from build123d import *

# Parameters (mm, degrees)
F0_W     = 130
F0_H     = 400
F0_R     = 5
F1_DEPTH = 4
F3_DEPTH = 5


with BuildPart() as f1:
    # F0 (on Right) → F1 (new body)
    with BuildSketch(Plane.YZ):
        with Locations((-28.497371, -1.37512)):
            Rectangle(F0_W, F0_H)
        with Locations((-63.497371, -21.37512)):
            Circle(F0_R, mode=Mode.SUBTRACT)
        with Locations((-13.497371, 168.62488)):
            Circle(F0_R, mode=Mode.SUBTRACT)
    extrude(amount=F1_DEPTH)

    # F2 (on face) → F3 (intersect)
    with BuildSketch(Plane.YZ):
        with BuildLine():
            ThreePointArc((-91.758037, 174.317055), (-76.660595, -2.275866), (-83.398097, -179.384868))
            ThreePointArc((-83.398097, -179.384868), (-78.326482, -194.79516), (-63.497371, -201.37512))
            Line((-63.497371, -201.37512), (-23.497371, -201.37512))
            ThreePointArc((-23.497371, -201.37512), (-11.939199, -197.69715), (-4.632088, -188.015985))
            ThreePointArc((-4.632088, -188.015985), (29.081884, -8.612485), (7.289094, 172.625817))
            ThreePointArc((7.289094, 172.625817), (1.908539, 181.642764), (-7.298468, 186.691201))
            ThreePointArc((-7.298468, 186.691201), (-38.508536, 193.035445), (-70.089166, 197.156317))
            ThreePointArc((-70.089166, 197.156317), (-86.482566, 191.010783), (-91.758037, 174.317055))
        make_face()
    extrude(amount=F3_DEPTH, mode=Mode.INTERSECT)


solid = f1.part
Work out the finished part from the listing and answer in its coordinate system (mm). Give positions to 0.01 mm unless a question says otherwise; leave off trailing zeros. Order: outer loops, then holes, each group sorted by start corner. A loop starts at its lowest first (then second) coordinate and runs counter-clockwise, first axis right, second up. Notation, with made-up numbers: (18, 86.5) -> (62, 86.5) arc R10 ccw to (62, 104.5) -> close; hole circle Ø9 at (31.25, 70). An arc over 180 degrees is marked (long way). Answer as a JSON object with one key per item and string values. Group by question number.
1. Section B-B on z = -36.5 is taken. Determine the outline of the cut face in (x, y).
2. Section C-C on z = 157.5 is taken. Determine the outline of the cut face in (x, y), plus the area to 3 significant figures.
3. Consider line 1 along Z through (x, y) = (2.9, -68); line 2 along Y through (x, z) = (1.25, 127.5); line 3 along Y through (x, z) = (2.8, -90.5). Determine where each line is inside the solid, lowest interval first. Write a range as [from, to].
4. A flat-ended cylindrical pin translates along its axis: pin 1 Ø13 at (y, z) = (-13.5, 168.62) entering from -X. Find the tip coordinate at first contact, or state that the pin passes through.
5. Section A-A on x = 1 is taken. Determine the outline of the cut face in (y, z).
6. The mould has two halves that part along Y. Classify faces 1 (the cylindrical face through (1.972, -68.493, -21.155)), 2 (the cylindrical face through (1.972, 2.015, 181.539)), 3 (the flat face through (4, -32, 1)): released by +Y, released by -Y, zero draft, split by the parting line, or undercut.
Result sheet:
{
 "1": {"outline": "(0, -76.26) -> (4, -76.26) -> (4, 27.51) -> (0, 27.51) -> close"},
 "2": {"outline": "(0, -89.37) -> (4, -89.37) -> (4, 11.3) -> (0, 11.3) -> close", "area": "403 mm^2"},
 "3": {"line 1": "z = [-200.86, -23.55], [-19.2, 196.95]", "line 2": "y = [-85.61, 18.03]", "line 3": "y = [-77.28, 20.73]"},
 "4": {"pin 1": "stops at x = 0"},
 "5": {"outline": "(-91.76, 174.32) arc R1438.26 cw to (-83.4, -179.38) arc R20 ccw to (-63.5, -201.38) -> (-23.5, -201.38) arc R20 ccw to (-4.63, -188.02) arc R600 ccw to (7.29, 172.63) arc R20 ccw to (-7.3, 186.69) arc R450 ccw to (-70.09, 197.16) arc R20 ccw to start; hole circle Ø10 at (-63.5, -21.38); hole circle Ø10 at (-13.5, 168.62)"},
 "6": {"face 1": "undercut", "face 2": "released by +Y", "face 3": "zero draft"}
}
